from build123d import *

# Parameters (mm, degrees)
SKETCH_1_W                  = 46
SKETCH_1_H                  = 37.9
EXTRUDE_1_DEPTH             = 4
HOLE_WIZARD_M4_1_AT_2_COUNT = 2
HOLE_WIZARD_M4_1_AT_2_PITCH = 38
SKETCH_5_W                  = 30
SKETCH_5_H                  = 31.9
CUT_EXTRUDE_1_DEPTH         = 19
SKETCH_6_W                  = 40
SKETCH_6_H                  = 17.9
CUT_EXTRUDE_2_DEPTH         = 34
FILLET_1_R                  = 1.6
FILLET_2_R                  = 1.5


with BuildPart() as part:
    # 草图1 → 凸台-拉伸1 (new, symmetric)
    with BuildSketch(Plane.XY):
        Rectangle(SKETCH_1_W, SKETCH_1_H)
    extrude(amount=EXTRUDE_1_DEPTH, both=True)

    # 草图4 → M4 螺纹孔1 (revolve, cut)
    with BuildSketch(Plane(origin=(-19, 18.95, 0), x_dir=(0, 0, 1), z_dir=(1, 0, 0))):
        Polygon((0, 0), (0, 9.591420021), (1.65, 8.6), (1.65, 0), align=None)
    hole_wizard_m4_1 = revolve(axis=Axis((-19, 25.3, 0), (0, -1, 0)), mode=Mode.SUBTRACT)

    # M4 螺纹孔1 at 2: M4 螺纹孔1 ×2
    with Locations(*[(i * HOLE_WIZARD_M4_1_AT_2_PITCH, 0, 0) for i in range(1, HOLE_WIZARD_M4_1_AT_2_COUNT)]):
        add(hole_wizard_m4_1, mode=Mode.SUBTRACT)

    # 镜向1: M4 螺纹孔1 across plane
    add(hole_wizard_m4_1.mirror(Plane.ZX), mode=Mode.SUBTRACT)

    # 镜向1 copy 1 sketch → 镜向1 copy 1 (revolve, cut)
    with BuildSketch(Plane(origin=(19, -18.95, 0), x_dir=(0, 0, 1), z_dir=(1, 0, 0))):
        Polygon((0, 0), (0, -9.591420021), (1.65, -8.6), (1.65, 0), align=None)
    revolve(axis=Axis((19, -25.3, 0), (0, -1, 0)), mode=Mode.SUBTRACT)

    # 草图5 → 切除-拉伸1 (cut, symmetric)
    with BuildSketch(Plane.XY.offset(4)):
        Rectangle(SKETCH_5_W, SKETCH_5_H)
    extrude(amount=CUT_EXTRUDE_1_DEPTH, both=True, mode=Mode.SUBTRACT)

    # 草图6 → 切除-拉伸2 (cut, symmetric)
    with BuildSketch(Plane.XY.offset(4)):
        Rectangle(SKETCH_6_W, SKETCH_6_H)
    extrude(amount=CUT_EXTRUDE_2_DEPTH, both=True, mode=Mode.SUBTRACT)

    # 圆角1
    fillet_1_edges = [part.edges().sort_by_distance(p)[0] for p in [
        (15, 15.95, 0),
        (15, -15.95, 0),
        (-15, -15.95, 0),
        (-15, 15.95, 0),
        (-15, 8.95, 0),
        (-15, -8.95, 0),
        (20, 8.95, 0),
        (-20, -8.95, 0),
        (20, -8.95, 0),
        (15, -8.95, 0),
        (15, 8.95, 0),
        (-20, 8.95, 0),
    ]]
    fillet(fillet_1_edges, radius=FILLET_1_R)

    # 圆角2
    fillet_2_edges = [part.edges().sort_by_distance(p)[0] for p in [
        (23, -18.95, 0),
        (-23, -18.95, 0),
        (-23, 18.95, 0),
        (23, 18.95, 0),
    ]]
    fillet(fillet_2_edges, radius=FILLET_2_R)


solid = part.part
Design review of the part built by this model. Coordinates are the model's own, in mm. A direction names the side the tool comes from. Coordinates: 2 decimals unless noted, no trailing zeros. Loops run counter-clockwise (first coordinate to the right, second up) from the corner with the lowest first, then second, coordinate; pieces in that order, holes last. Notation, with made-up numbers: (74, 19) - (126, 19) arc R21 ccw to (126, 49) - close; hole circle Ø5 at (-0.75, 68.25). An arc over 180 degrees is marked (long way). Use CSV: the item, a comma, the result in double quotes. Start each with the question number.
1. To check wall thickness, follow probe 1 along X at (y, z) = (13.5, 0); probe 2 along Z at (x, y) = (19, -16.5); probe 3 along Y at (x, z) = (4.5, 3.75). State the ranges of each line that lie inside material, in increasing order.
2. Mouldability with a two-part tool opening along Z and no side actions: class faces 1 (the cylindrical face through (-19.54, -8.47, 0.06)), 2 (the cylindrical face through (-20.636, 14.71, -0.215)), 3 (the flat face through (0, -17, -4)) as released by +Z, released by -Z, zero draft, split by the parting line, or undercut.
3. For faces 4 (the cylindrical face through (17.364, -14.71, -0.215)), 5 (the conical face through (18.72, 9.53, -0.04)), 6 (the cylindrical face through (15.46, -9.43, -0.06)), list the 3-axis set-ups (+Z, -Z, +X, -X, +Y, -Y) from which the entire face can be reached by the end or side of a thin tool; tool diameter is ignored.
4. Clearance check with flat-ended pins moving along their axes: pin 1 (2 mm diameter, centred on x = -19, z = 0, fed in from -Y); pin 2 (3 mm diameter, centred on x = -17, y = -5, fed in from -Z). State where each tip first meets the part, or that it passes through.
5. Add section D-D on y = 3. Give the boundary of the cut face in (x, z), plus the area to 3 significant figures.
6. Add section A-A on y = 11.5. Give the boundary of the cut face in (x, z).
7. Add section B-B on x = -12. Give the boundary of the cut face in (y, z).
Resolved:
1,probe 1,"-23 to -20.65, -17.35 to -15, 15 to 17.35, 20.65 to 23"
1,probe 2,"-4 to -1.65, 1.65 to 4"
1,probe 3,"-18.95 to -15.95, 15.95 to 18.95"
2,face 1,"zero draft"
2,face 2,"undercut"
2,face 3,"released by -Z"
3,face 4,"-Y"
3,face 5,"+Y"
3,face 6,"+Z, -Z"
4,pin 1,"y = -9.96"
4,pin 2,"through"
5,outline,"(-23, -4) - (-20, -4) - (-20, 4) - (-23, 4) - close; (20, -4) - (23, -4) - (23, 4) - (20, 4) - close"
5,area,"48.0 mm2"
6,outline,"(-23, -4) - (-15, -4) - (-15, 4) - (-23, 4) - close; (15, -4) - (23, -4) - (23, 4) - (15, 4) - close; hole circle Ø3.3 at (-19, 0); hole circle Ø3.3 at (19, 0)"
7,outline,"(-18.95, -4) - (-15.95, -4) - (-15.95, 4) - (-18.95, 4) - close; (15.95, -4) - (18.95, -4) - (18.95, 4) - (15.95, 4) - close"
